Work out the finished part from the listing and answer in its coordinate system (mm). Give positions to 0.01 mm unless a question says otherwise; leave off trailing zeros. Order: outer loops, then holes, each group sorted by start corner. A loop starts at its lowest first (then second) coordinate and runs counter-clockwise, first axis right, second up.
```python
from build123d import *

# Parameters (mm, degrees)
BOX_W     = 20
BOX_H     = 30
BOX_DEPTH = 3
PAD_DEPTH = 5
FILLET_R  = 2


with BuildPart() as cubo:
    # Box → Box (new body)
    with BuildSketch(Plane(origin=(-55, -27, -3), x_dir=(1, 0, 0), z_dir=(0, 0, 1))):
        with Locations((10, 15)):
            Rectangle(BOX_W, BOX_H)
    extrude(amount=BOX_DEPTH)


with BuildPart() as fillet_body:
    # Sketch → Pad (new body)
    with BuildSketch(Plane.XY):
        Polygon((48.214441, 18.44022), (48.214441, -46.55978), (-21.785559, -46.55978), (-30.548117, -55.842846), (-50.548117, -55.842846), (-60.130928, -45.949108), (-60.130928, 19.287283), (-49.72015, 28.44022), (-29.72015, 28.44022), (-21.785559, 18.44022), align=None)
    extrude(amount=PAD_DEPTH)

    # Fusion: union Cubo
    add(cubo.part)

    # Fillet
    fillet_edges = [fillet_body.edges().sort_by_distance(p)[0] for p in [
        (48.214441, 18.44022, 2.5),
        (48.214441, -46.55978, 2.5),
    ]]
    fillet(fillet_edges, radius=FILLET_R)


solid = fillet_body.part
```
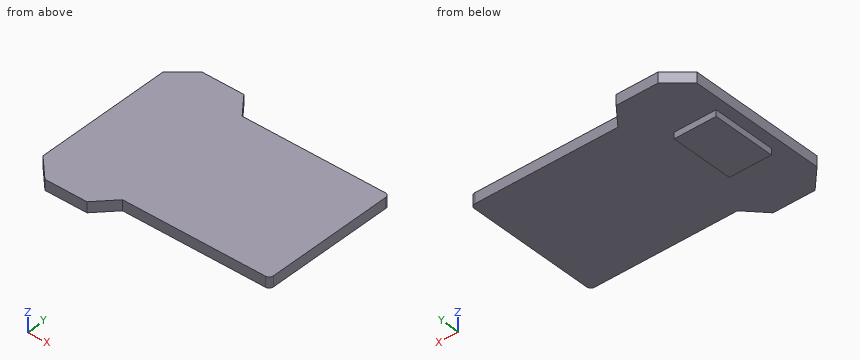
1. The part is cut by section B-B (z = 1.75). Write down the section's boundary in (x, y), then the cut area to 3 significant figures.
Findings below:
outline: (-60.13, -45.95) - (-50.55, -55.84) - (-30.55, -55.84) - (-21.79, -46.56) - (46.21, -46.56) arc R2 ccw to (48.21, -44.56) - (48.21, 16.44) arc R2 ccw to (46.21, 18.44) - (-21.79, 18.44) - (-29.72, 28.44) - (-49.72, 28.44) - (-60.13, 19.29) - close
area: 7,600 mm2
2. The part is cut by section D-D (x = 11.5). Write down the section's boundary in (y, z), then the cut area to 3 significant figures.
Findings below:
outline: (-46.56, 0) - (18.44, 0) - (18.44, 5) - (-46.56, 5) - close
area: 325 mm2
3. The part is cut by section C-C (y = 11). Write down the section's boundary in (x, z), then the cut area to 3 significant figures.
Findings below:
outline: (-60.13, 0) - (48.21, 0) - (48.21, 5) - (-60.13, 5) - close
area: 542 mm2
4. The part is cut by section A-A (x = -39). Write down the section's boundary in (y, z), then the cut area to 3 significant figures.
Findings below:
outline: (-55.84, 0) - (-27, 0) - (-27, -3) - (3, -3) - (3, 0) - (28.44, 0) - (28.44, 5) - (-55.84, 5) - close
area: 511 mm2
5. Given P1, Ø2, axis at x = 16, z = 1.5, coming from the +Y side; P2, Ø1, axis at y = -28.5, z = -2, coming from the -X side; P3, Ø1.5, axis at x = 18, z = 2.5, coming from the -Y side; P4, Ø8, axis at x = -4.5, y = -31, coming from the -Z side, each flat-ended and moving along its own axis, determine where each tip first touches the part or whether it passes through.
Findings below:
P1: stops at y = 18.44
P2: passes through
P3: stops at y = -46.56
P4: stops at z = 0
6. Straight lines are drawn through the part: probe 1 along Z at (x, y) = (8, -35); probe 2 along X at (y, z) = (-13, -0.5); probe 3 along Y at (x, z) = (-4, 4.25). For each, find the intervals that lie inside material, in ascending order.
Findings below:
probe 1: z = 0 to 5
probe 2: x = -55 to -35
probe 3: y = -46.56 to 18.44
